```python
from build123d import *

# Parameters (mm, degrees)
SKETCH1_R           = 15
SKETCH1_R_2         = 1.5
BOSS_EXTRUDE1_DEPTH = 4
SKETCH2_R           = 1
CUT_EXTRUDE1_DEPTH  = 4


with BuildPart() as part:
    # Sketch1 → Boss-Extrude1 (new body)
    with BuildSketch(Plane.XY):
        with BuildLine():
            Line((12.191311906, -32.739139882), (13.561737619, -34.452172024))
            ThreePointArc((13.561737619, -34.452172024), (13.887256638, -35.039548236), (14, -35.701562119))
            Line((14, -35.701562119), (14, -43))
            ThreePointArc((14, -43), (13.414213562, -44.414213562), (12, -45))
            Line((12, -45), (-12.018212743, -45))
            ThreePointArc((-12.018212743, -45), (-13.432426305, -44.414213562), (-14.018212743, -43))
            Line((-14.018212743, -43), (-14.018212743, -35.691034212))
            ThreePointArc((-14.018212743, -35.691034212), (-13.905469381, -35.029020329), (-13.579950362, -34.441644117))
            Line((-13.579950362, -34.441644117), (-12.209524648, -32.728611975))
            ThreePointArc((-12.209524648, -32.728611975), (-10.581929551, -29.791730914), (-10.018212743, -26.481661499))
            Line((-10.018212743, -26.481661499), (-10.018212743, -17.309980169))
            ThreePointArc((-10.018212743, -17.309980169), (0.010518327, 19.999997234), (10, -17.320508076))
            Line((10, -17.320508076), (10, -26.492189406))
            ThreePointArc((10, -26.492189406), (10.563716808, -29.802258821), (12.191311906, -32.739139882))
        make_face()
        Circle(SKETCH1_R, mode=Mode.SUBTRACT)
        with Locations((0, 17.5)):
            Circle(SKETCH1_R_2, mode=Mode.SUBTRACT)
        with Locations((15.155444566, -8.75)):
            Circle(SKETCH1_R_2, mode=Mode.SUBTRACT)
        with Locations((-15.155444566, -8.75)):
            Circle(SKETCH1_R_2, mode=Mode.SUBTRACT)
        with BuildLine():
            Line((-3, -19), (-3, -33.13932584))
            ThreePointArc((-3, -33.13932584), (-5, -35.13932584), (-7, -33.13932584))
            Line((-7, -33.13932584), (-7, -19))
            ThreePointArc((-7, -19), (-5, -17), (-3, -19))
        make_face(mode=Mode.SUBTRACT)
        with BuildLine():
            Line((3, -19), (3, -33.13932584))
            ThreePointArc((3, -33.13932584), (5, -35.13932584), (7, -33.13932584))
            Line((7, -33.13932584), (7, -19))
            ThreePointArc((7, -19), (5, -17), (3, -19))
        make_face(mode=Mode.SUBTRACT)
    extrude(amount=BOSS_EXTRUDE1_DEPTH)

    # Sketch2 → Cut-Extrude1 (cut)
    with BuildSketch(Plane.XZ.offset(45)):
        with Locations((-10.009106371, 2)):
            Circle(SKETCH2_R)
        with Locations((9.990893629, 2)):
            Circle(SKETCH2_R)
    extrude(amount=-CUT_EXTRUDE1_DEPTH, mode=Mode.SUBTRACT)


solid = part.part
```
For this review, take the finished solid that the model builds, in its own axes (mm). A direction names the side the tool comes from. Coordinates: 2 decimals unless noted, no trailing zeros. Write each loop counter-clockwise with the first axis right and the second up, starting at its lowest first coordinate (ties: lowest second). Pieces come first, ordered by that corner, then holes.
(1) Wall thickness on probe 1 along Y at (x, z) = (0, 1.15); probe 2 along X at (y, z) = (-25, 0.6); probe 3 along Y at (x, z) = (6.5, 1.2): over which ranges is each line inside the solid? List them lowest first.
(2) Add section D-D on y = 0. Give the boundary of the cut face in (x, z), then the cut area to 3 significant figures.
(3) Add section A-A on x = 0. Give the boundary of the cut face in (y, z), then the cut area to 3 significant figures.
(4) For pin 1 Ø1.2 at (y, z) = (-22.5, 2) entering from -X; pin 2 Ø1.2 at (y, z) = (-26.5, 1.5) entering from +X; pin 3 Ø1.8 at (x, z) = (-10.01, 2) entering from -Y; pin 4 Ø18 at (x, y) = (0, 0) entering from -Z, all flat-tipped, find the tip position at first contact; note any pin that passes through.
(5) Add section B-B on y = -13.5. Give the boundary of the cut face in (x, z), then the cut area to 3 significant figures.
(6) The part is to be moulded in two halves that separate along X. For faces 1 (the face through (-13.91, -35.04, 1.97)), 2 (the face through (13.884, -35.031, 1.972)), 3 (the face through (-14.985, 0.66, 1.972)), say which applies: +X half, -X half, draft (parallel to the pull), parting line (faces both ways), or undercut.
(7) Tool access review of faces 4 (the face through (14, -39, 2)), 5 (the face through (-11.01, -43.03, 2.04)), 6 (the face through (12.867, -33.584, 1.972)), 7 (the face through (-7, -26, 2)): name each direction out of +Z, -Z, +X, -X, +Y, -Y from which nothing blocks a thin tool from reaching the whole face with its end or side.
(8) Add section C-C on y = -23.5. Give the boundary of the cut face in (x, z), then the cut area to 3 significant figures.
Answer sheet:
1. probe 1: y = -45 to -15, 15 to 16, 19 to 20
1. probe 2: x = -10.02 to -7, -3 to 3, 7 to 10
1. probe 3: y = -45 to -34.46, -17.68 to -13.52, 13.52 to 18.91
2. outline: (-20, 0) - (-15, 0) - (-15, 4) - (-20, 4) - close; (15, 0) - (20, 0) - (20, 4) - (15, 4) - close
2. area: 40.0 mm2
3. outline: (-45, 0) - (-15, 0) - (-15, 4) - (-45, 4) - close; (15, 0) - (16, 0) - (16, 4) - (15, 4) - close; (19, 0) - (20, 0) - (20, 4) - (19, 4) - close
3. area: 128 mm2
4. pin 1: stops at x = -10.02
4. pin 2: stops at x = 10.02
4. pin 3: stops at y = -41
4. pin 4: passes through
5. outline: (-14.76, 0) - (-6.54, 0) - (-6.54, 4) - (-14.76, 4) - close; (6.54, 0) - (14.76, 0) - (14.76, 4) - (6.54, 4) - close
5. area: 65.7 mm2
6. face 1: -X half
6. face 2: +X half
6. face 3: undercut
7. face 4: +Z, -Z, +X, -Y
7. face 5: -Y
7. face 6: +Z, -Z, +X
7. face 7: +Z, -Z
8. outline: (-10.02, 0) - (-7, 0) - (-7, 4) - (-10.02, 4) - close; (-3, 0) - (3, 0) - (3, 4) - (-3, 4) - close; (7, 0) - (10, 0) - (10, 4) - (7, 4) - close
8. area: 48.1 mm2
